Print and shaded views of the part. All mm, measured from the part's lowest x, y and z. Give positions to 0.01 mm unless a question says otherwise; leave off trailing zeros. Loops run counter-clockwise (first coordinate to the right, second up) from the corner with the lowest first, then second, coordinate; pieces in that order, holes last. Notation, with made-up numbers: (49, 21) - (94, 21) arc R19 ccw to (94, 53) - close; hole circle Ø8 at (63, -20.75). An arc over 180 degrees is marked (long way). Return JSON: item names as keys, results as strings.
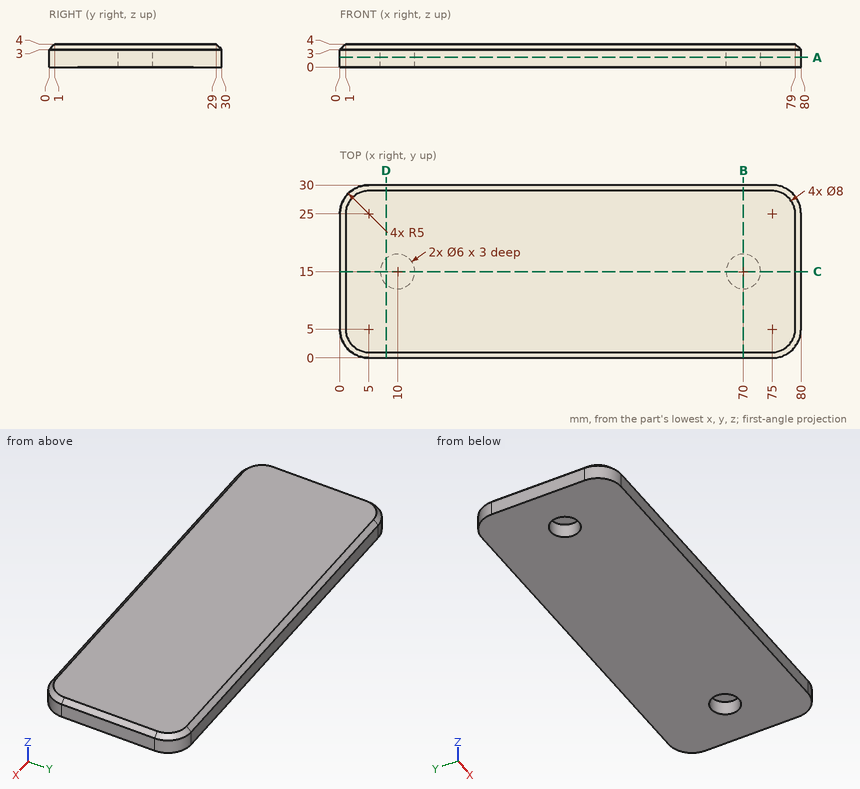
1. Cut at B-B, the plane x = 70. Write the cut outline in (y, z).
Values follow:
{"outline": "(0, 0) - (12, 0) - (12, 3) - (18, 3) - (18, 0) - (30, 0) - (30, 3) - (29, 4) - (1, 4) - (0, 3) - close"}
2. Drop flat-ended pins along their axis: P1, Ø5, axis at x = 68.5, y = 15.5, coming from the -Z side; P2, Ø2, axis at y = 3.5, z = 2, coming from the -X side; P3, Ø1.8, axis at x = 10.5, y = 14, coming from the -Z side. Give the stop position or say it passes through.
Values follow:
{"P1": "stops at z = 0", "P2": "stops at x = 0.03", "P3": "stops at z = 3"}
3. Cut at A-A, the plane z = 1.7. Write the cut outline in (x, y), plus the area to 3 significant figures.
Values follow:
{"outline": "(0, 5) arc R5 ccw to (5, 0) - (75, 0) arc R5 ccw to (80, 5) - (80, 25) arc R5 ccw to (75, 30) - (5, 30) arc R5 ccw to (0, 25) - close; hole circle Ø6 at (10, 15); hole circle Ø6 at (70, 15)", "area": "2,320 mm²"}
4. Cut at C-C, the plane y = 15. Write the cut outline in (x, z).
Values follow:
{"outline": "(0, 0) - (7, 0) - (7, 3) - (13, 3) - (13, 0) - (67, 0) - (67, 3) - (73, 3) - (73, 0) - (80, 0) - (80, 3) - (79, 4) - (1, 4) - (0, 3) - close"}
5. Cut at D-D, the plane x = 8. Write the cut outline in (y, z).
Values follow:
{"outline": "(0, 0) - (12.76, 0) - (12.76, 3) - (17.24, 3) - (17.24, 0) - (30, 0) - (30, 3) - (29, 4) - (1, 4) - (0, 3) - close"}
6. Drill centre lines: probe 1 along X at (y, z) = (15, 0.9); probe 2 along Y at (x, z) = (70, 2.05); probe 3 along Y at (x, z) = (7.5, 0.65). Where is each one in solid material? Low to high.
Values follow:
{"probe 1": "x = 0 to 7, 13 to 67, 73 to 80", "probe 2": "y = 0 to 12, 18 to 30", "probe 3": "y = 0 to 13.34, 16.66 to 30"}
